from build123d import *

# Parameters (mm, degrees)
MAIN_SHAPE_DEPTH                            = 6.35
FILLET1_R                                   = 3
F_3_48_TAPPED_HOLE1_D                       = 1.9939
F_3_48_TAPPED_HOLE1_DEPTH                   = 6.61
F_3_48_TAPPED_HOLE1_TIP                     = 0.599027994
F_3_48_TAPPED_HOLE1_FOR_ARDUINO_MOUNT_D     = 2.0828
F_3_48_TAPPED_HOLE1_FOR_ARDUINO_MOUNT_DEPTH = 7.3
F_3_48_TAPPED_HOLE1_FOR_ARDUINO_MOUNT_TIP   = 0.625736249


with BuildPart() as part:
    # Sketch1 → main shape (new body)
    with BuildSketch(Plane.XY):
        Polygon((0, 0), (0, 100), (21.818, 100), (21.818, 80), (61.818, 80), (61.818, 100), (83.636, 100), (83.636, 0), (71.136, 0), (71.136, 25.68), (66.818, 25.68), (66.818, 0), (16.818, 0), (16.818, 25.68), (12.5, 25.68), (12.5, 0), align=None)
    extrude(amount=MAIN_SHAPE_DEPTH)

    # Fillet1
    fillet1_edges = [part.edges().sort_by_distance(p)[0] for p in [
        (0, 100, 3.175),
        (21.818, 100, 3.175),
        (61.818, 100, 3.175),
        (83.636, 100, 3.175),
    ]]
    fillet(fillet1_edges, radius=FILLET1_R)

    # #3-48 Tapped Hole1
    with Locations(Plane.XY.offset(6.35)):
        with Locations((17.818, 95), (17.818, 86), (65.818, 86), (65.818, 95)):
            Hole(F_3_48_TAPPED_HOLE1_D / 2, depth=F_3_48_TAPPED_HOLE1_DEPTH)
            with Locations((0, 0, -(F_3_48_TAPPED_HOLE1_DEPTH + F_3_48_TAPPED_HOLE1_TIP / 2))):  # 118° drill point
                Cone(0, F_3_48_TAPPED_HOLE1_D / 2, F_3_48_TAPPED_HOLE1_TIP, mode=Mode.SUBTRACT)

    # #3-48 Tapped Hole1 for arduino mount
    with Locations(Plane.XY.offset(6.35)):
        with Locations((21.3, 75), (20, 26.9), (73.4, 26.9), (73.4, 59.8), (10.236, 31.9), (63.636, 26.9), (62.336, 75), (10.811692828, 59.393923536)):
            Hole(F_3_48_TAPPED_HOLE1_FOR_ARDUINO_MOUNT_D / 2, depth=F_3_48_TAPPED_HOLE1_FOR_ARDUINO_MOUNT_DEPTH)
            with Locations((0, 0, -(F_3_48_TAPPED_HOLE1_FOR_ARDUINO_MOUNT_DEPTH + F_3_48_TAPPED_HOLE1_FOR_ARDUINO_MOUNT_TIP / 2))):  # 118° drill point
                Cone(0, F_3_48_TAPPED_HOLE1_FOR_ARDUINO_MOUNT_D / 2, F_3_48_TAPPED_HOLE1_FOR_ARDUINO_MOUNT_TIP, mode=Mode.SUBTRACT)


solid = part.part
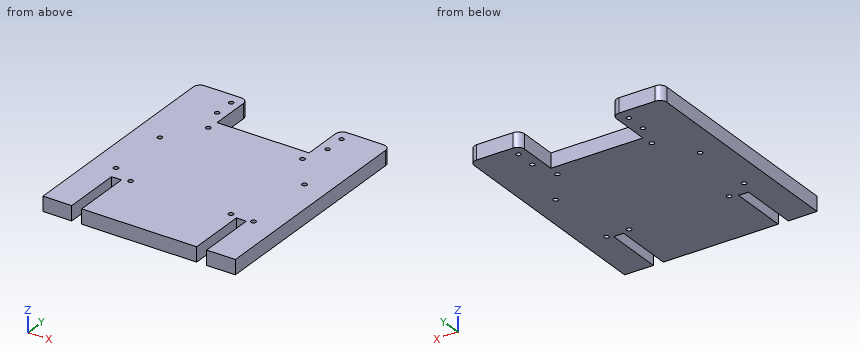
Read the model definition and answer for the solid it produces. Units are mm, in the model's axes. Coordinates: 2 decimals unless noted, no trailing zeros. Order: outer loops, then holes, each group sorted by start corner. A loop starts at its lowest first (then second) coordinate and runs counter-clockwise, first axis right, second up. Notation, with made-up numbers: (59.25, -36.5) -> (80.25, -36.5) arc R15 cw to (80.25, -18.5) -> close; hole circle Ø5 at (-18.75, 89). An arc over 180 degrees is marked (long way). Answer as a JSON object with one key per item and string values.
1) Consider line 1 along X through (y, z) = (75, 3.75); line 2 along Y through (x, z) = (18, 3.5); line 3 along X through (y, z) = (25.5, 3). Determine where each line is inside the solid, lowest interval first. Write a range as from..to.
Model answer:
{"line 1": "x = 0..20.26, 22.34..61.29, 63.38..83.64", "line 2": "y = 0..85.02, 86.98..94.02, 95.98..100", "line 3": "x = 0..12.5, 16.82..66.82, 71.14..83.64"}
2) A cutting plane is placed at B-B, the plane z = 5. State how many separate pieces and enclosed holes the cut face has, plus the area to 3 significant figures.
Model answer:
{"separate pieces": "1", "enclosed holes": "12", "area": "7,290 mm²"}
3) A cutting plane is placed at A-A, the plane y = 6.5. Determine the outline of the cut face in (x, z).
Model answer:
{"outline": "(0, 0) -> (12.5, 0) -> (12.5, 6.35) -> (0, 6.35) -> close; (16.82, 0) -> (66.82, 0) -> (66.82, 6.35) -> (16.82, 6.35) -> close; (71.14, 0) -> (83.64, 0) -> (83.64, 6.35) -> (71.14, 6.35) -> close"}
4) A cutting plane is placed at C-C, the plane x = 15.5. Determine the outline of the cut face in (y, z).
Model answer:
{"outline": "(25.68, 0) -> (100, 0) -> (100, 6.35) -> (25.68, 6.35) -> close"}
5) Each of these flat-tipped pins is pushed along its axis until it touches: pin 1 (2 mm diameter, centred on x = 68, z = 4, fed in from -Y); pin 2 (1.9 mm diameter, centred on x = 35.5, z = 3.5, fed in from +Y). Where does it stop, or does it pass through?
Model answer:
{"pin 1": "stops at y = 25.68", "pin 2": "stops at y = 80"}
